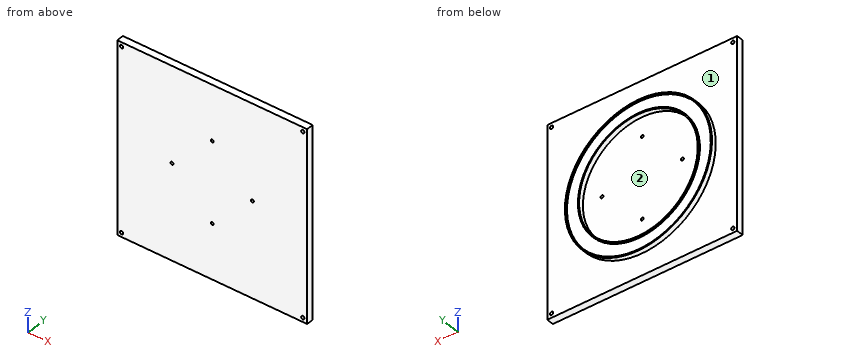
from build123d import *

# Parameters (mm, degrees)
SKETCH1_W           = 800
SKETCH1_H           = 800
BOSS_EXTRUDE1_DEPTH = 15
SKETCH4_R           = 6
CUT_EXTRUDE3_DEPTH  = 567.480361531
SKETCH3_R           = 310
SKETCH3_R_2         = 250
BOSS_EXTRUDE2_DEPTH = 20
SKETCH5_R           = 305
SKETCH5_R_2         = 255
CUT_EXTRUDE4_DEPTH  = 5
SKETCH6_R           = 7
CUT_EXTRUDE5_DEPTH  = 567.480361531


with BuildPart() as part:
    # Sketch1 → Boss-Extrude1 (new, symmetric)
    with BuildSketch(Plane(origin=(0, 0, 0), x_dir=(1, 0, 0), z_dir=(0, 1, 0))):
        Rectangle(SKETCH1_W, SKETCH1_H)
    extrude(amount=BOSS_EXTRUDE1_DEPTH, both=True)

    # Sketch4 → Cut-Extrude3 (cut, through all)
    with BuildSketch(Plane(origin=(0, 15, 0), x_dir=(1, 0, 0), z_dir=(0, 1, 0))):
        with Locations(Location((0, 169.5, 0), (0, 0, 270))):
            Circle(SKETCH4_R)
        with Locations(Location((169.5, 0, 0), (0, 0, 270))):
            Circle(SKETCH4_R)
        with Locations(Location((0, -169.5, 0), (0, 0, 90))):
            Circle(SKETCH4_R)
        with Locations(Location((-169.5, 0, 0), (0, 0, 90))):
            Circle(SKETCH4_R)
    extrude(amount=-CUT_EXTRUDE3_DEPTH, mode=Mode.SUBTRACT)

    # Sketch3 → Boss-Extrude2 (add)
    with BuildSketch(Plane(origin=(0, 15, 0), x_dir=(1, 0, 0), z_dir=(0, 1, 0))):
        with Locations(Location((0, 0, 0), (0, 0, 270))):
            Circle(SKETCH3_R)
        with Locations(Location((0, 0, 0), (0, 0, 270))):
            Circle(SKETCH3_R_2, mode=Mode.SUBTRACT)
    extrude(amount=BOSS_EXTRUDE2_DEPTH)

    # Sketch5 → Cut-Extrude4 (cut)
    with BuildSketch(Plane(origin=(0, 35, 0), x_dir=(1, 0, 0), z_dir=(0, 1, 0))):
        with Locations(Location((0, 0, 0), (0, 0, 270))):
            Circle(SKETCH5_R)
        with Locations(Location((0, 0, 0), (0, 0, 270))):
            Circle(SKETCH5_R_2, mode=Mode.SUBTRACT)
    extrude(amount=-CUT_EXTRUDE4_DEPTH, mode=Mode.SUBTRACT)

    # Sketch6 → Cut-Extrude5 (cut, through all)
    with BuildSketch(Plane(origin=(0, 15, 0), x_dir=(1, 0, 0), z_dir=(0, 1, 0))):
        with Locations(Location((-382, 382, 0), (0, 0, 270))):
            Circle(SKETCH6_R)
        with Locations(Location((382, 382, 0), (0, 0, 90))):
            Circle(SKETCH6_R)
        with Locations(Location((382, -382, 0), (0, 0, 270))):
            Circle(SKETCH6_R)
        with Locations(Location((-382, -382, 0), (0, 0, 90))):
            Circle(SKETCH6_R)
    extrude(amount=-CUT_EXTRUDE5_DEPTH, mode=Mode.SUBTRACT)


solid = part.part
For this review, take the finished solid that the model builds, in its own axes (mm). Face numbers are marked on the shaded views. Round coordinates to 2 decimals unless told otherwise and drop trailing zeros. Loops run counter-clockwise (first coordinate to the right, second up) from the corner with the lowest first, then second, coordinate; pieces in that order, holes last. Notation, with made-up numbers: (44, -7) - (65, -7) arc R28 cw to (65, 26) - close; hole circle Ø10 at (65.25, 59). An arc over 180 degrees is marked (long way). One line per item, written item: value. Start each with the question number.
Item 1: Take a section at A-A (x = 81.5). Give the boundary of the cut face in (y, z), plus the area to 3 significant figures.
Item 2: Clearance check with flat-ended pins moving along their axes: pin 1 Ø10 at (x, z) = (-132.5, -68.5) entering from +Y; pin 2 Ø4 at (y, z) = (22.5, 125) entering from +X; pin 3 Ø10 at (x, y) = (265, 23) entering from +Z. State where each tip first meets the part, or that it passes through.
Item 3: The part is to be moulded in two halves that separate along Z. For the marked faces 1 and 2, say which applies: +Z half, -Z half, draft (parallel to the pull), parting line (faces both ways), or undercut.
Item 4: Take a section at B-B (z = -60.5). Give the boundary of the cut face in (x, y).
Item 5: For L1, parallel to X at y = 8.25, z = 382; L2, parallel to X at y = 5.25, z = 0, list the stretches that pass through material, from the lowest coordinate up.
Answer below:
1. outline: (-15, -400) - (15, -400) - (15, -299.09) - (35, -299.09) - (35, -293.91) - (30, -293.91) - (30, -241.63) - (35, -241.63) - (35, -236.34) - (15, -236.34) - (15, 236.34) - (35, 236.34) - (35, 241.63) - (30, 241.63) - (30, 293.91) - (35, 293.91) - (35, 299.09) - (15, 299.09) - (15, 400) - (-15, 400) - close
1. area: 26,000 mm2
2. pin 1: stops at y = 15
2. pin 2: stops at x = 284.55
2. pin 3: stops at z = 168.82
3. face 1: draft
3. face 2: undercut
4. outline: (-400, -15) - (400, -15) - (400, 15) - (304.04, 15) - (304.04, 35) - (298.94, 35) - (298.94, 30) - (247.72, 30) - (247.72, 35) - (242.57, 35) - (242.57, 15) - (-242.57, 15) - (-242.57, 35) - (-247.72, 35) - (-247.72, 30) - (-298.94, 30) - (-298.94, 35) - (-304.04, 35) - (-304.04, 15) - (-400, 15) - close
5. L1: x = -400 to -389, -375 to 375, 389 to 400
5. L2: x = -400 to -175.5, -163.5 to 163.5, 175.5 to 400
